For this review, use the dimensioned drawing (mm, ordinates from the lowest corner) and the shaded views. Round coordinates to 2 decimals unless told otherwise and drop trailing zeros. Write each loop counter-clockwise with the first axis right and the second up, starting at its lowest first coordinate (ties: lowest second). Pieces come first, ordered by that corner, then holes. Notation, with made-up numbers: M 85,-9 L 139,-9 A17 ccw 139,9 Z; hole C 38,88.5 d4. An arc over 180 degrees is marked long. Use one line per item in the form item = value. Start each with the question number.
Item 1: Add section C-C (z = 1.8). Count the separate pieces of the cut face and the enclosed holes in it, and give its area (3 significant figures).
Item 2: Add section B-B (x = 285). State the section outline as (y, z) points.
Item 3: Add section A-A (y = 15). State the section outline as (x, z) points.
Item 4: For line 1 (Y direction, x = 15, z = 2.45); line 2 (X direction, y = 41.5, z = 1.45); line 3 (X direction, y = 17, z = 0.9) (1 decimal), list the stretches that pass through material, from the lowest coordinate up. Write a range as [from, to].
Item 5: For P1, Ø7.5, axis at x = 15, y = 15, coming from the -Z side, flat-tipped, find the tip position at first contact; note if it passes through.
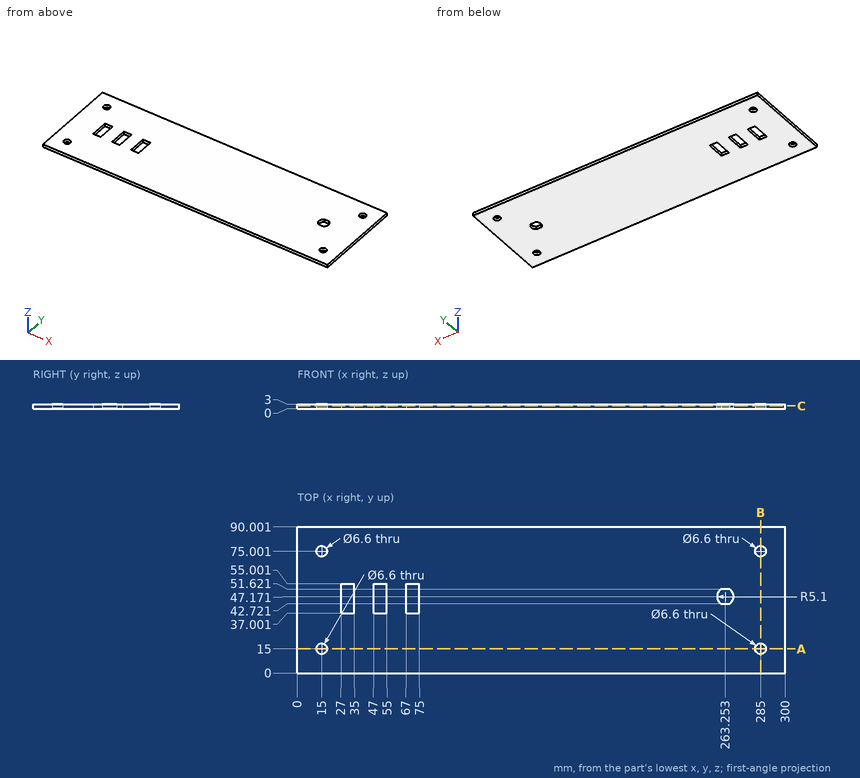
Calculated:
q1.separate_pieces = 1
q1.enclosed_holes = 8
q1.area = 26,400 mm^2
q2.outline = M 0,0 L 11.7,0 L 11.7,3 L 0,3 Z; M 18.3,0 L 71.7,0 L 71.7,3 L 18.3,3 Z; M 78.3,0 L 90,0 L 90,3 L 78.3,3 Z
q3.outline = M 0,0 L 11.7,0 L 11.7,3 L 0,3 Z; M 18.3,0 L 281.7,0 L 281.7,3 L 18.3,3 Z; M 288.3,0 L 300,0 L 300,3 L 288.3,3 Z
q4.line_1 = [0, 11.7], [18.3, 71.7], [78.3, 90]
q4.line_2 = [0, 27], [35, 47], [55, 67], [75, 300]
q4.line_3 = [0, 12.4], [17.6, 282.4], [287.6, 300]
q5.P1 = 0
